For this review, take the finished solid that the model builds, in its own axes (mm). Coordinates: 2 decimals unless noted, no trailing zeros. Order: outer loops, then holes, each group sorted by start corner. A loop starts at its lowest first (then second) coordinate and runs counter-clockwise, first axis right, second up. Notation, with made-up numbers: (77.25, 73.25) -> (99.25, 73.25) arc R30 ccw to (99.25, 105.25) -> close; hole circle Ø4 at (10.5, -11). An arc over 180 degrees is marked (long way). Return JSON: item names as keys, results as strings. Group by question number.
Item 1: Take a section at D-D (x = 7.5). Write out the cut boundary in (y, z).
Item 2: For line 1 along Y through (x, z) = (22.5, -9.75); line 2 along X through (y, z) = (9, -10); line 3 along Y through (x, z) = (21.75, -9.5), list the stretches that pass through material, from the lowest coordinate up.
Item 3: Take a section at B-B (y = 10). Write out the cut boundary in (x, z), then the cut area to 3 significant figures.
Item 4: Insertion check: pin 1 (5 mm diameter, centred on x = 19.5, y = 8, fed in from +Z). The pin has a flat end and moves straight along its axis. Give the tip position at first contact, or say it passes through.
Item 5: Take a section at A-A (z = -20). Write out the cut boundary in (x, y).
Item 6: Take a section at C-C (x = 22.5). Write out the cut boundary in (y, z), then the cut area to 3 significant figures.
Item 7: Draft analysis for pull direction X (two halves, no side actions). For faces 1 (the flat face through (15, 20, -15)), 2 (the flat face through (0, 10, -15)), 3 (the cylindrical face through (5.94, 9.86, -20.35)), 4 (the flat face through (30, 10, -15)), state which applies: +X half, -X half, draft (parallel to the pull), parting line (faces both ways), or undercut.
```python
from build123d import *

# Parameters (mm, degrees)
SKETCH_1_W          = 30
SKETCH_1_H          = 30
SKETCH_1_R          = 1.6
EXTRUDE_1_DEPTH     = 20
SKETCH_2_R          = 1.6
CUT_EXTRUDE_1_DEPTH = 47.904157598


with BuildPart() as part:
    # 草图1 → 凸台-拉伸1 (new body)
    with BuildSketch(Plane(origin=(0, 0, 0), x_dir=(1, 0, 0), z_dir=(0, 1, 0))):
        with Locations((15, 15)):
            Rectangle(SKETCH_1_W, SKETCH_1_H)
        with Locations(Location((7.5, 20, 0), (0, 0, 270))):
            Circle(SKETCH_1_R, mode=Mode.SUBTRACT)
        with Locations(Location((7.5, 10, 0), (0, 0, 270))):
            Circle(SKETCH_1_R, mode=Mode.SUBTRACT)
    extrude(amount=EXTRUDE_1_DEPTH)

    # 草图2 → 切除-拉伸1 (cut, through all)
    with BuildSketch(Plane(origin=(0, 0, -30), x_dir=(-1, 0, 0), z_dir=(0, 0, -1))):
        with Locations((-22.5, 10)):
            Circle(SKETCH_2_R)
    extrude(amount=-CUT_EXTRUDE_1_DEPTH, mode=Mode.SUBTRACT)


solid = part.part
```
Findings below:
{
 "1": {"outline": "(0, -30) -> (20, -30) -> (20, -21.6) -> (0, -21.6) -> close; (0, -18.4) -> (20, -18.4) -> (20, -11.6) -> (0, -11.6) -> close; (0, -8.4) -> (20, -8.4) -> (20, 0) -> (0, 0) -> close"},
 "2": {"line 1": "y = 0 to 8.4, 11.6 to 20", "line 2": "x = 0 to 5.9, 9.1 to 21.25, 23.75 to 30", "line 3": "y = 0 to 8.59, 11.41 to 20"},
 "3": {"outline": "(0, -30) -> (20.9, -30) -> (20.9, 0) -> (0, 0) -> close; (24.1, -30) -> (30, -30) -> (30, 0) -> (24.1, 0) -> close; hole circle Ø3.2 at (7.5, -20); hole circle Ø3.2 at (7.5, -10)", "area": "788 mm2"},
 "4": {"pin 1": "stops at z = 0"},
 "5": {"outline": "(0, 0) -> (5.9, 0) -> (5.9, 20) -> (0, 20) -> close; (9.1, 0) -> (30, 0) -> (30, 20) -> (9.1, 20) -> close; hole circle Ø3.2 at (22.5, 10)"},
 "6": {"outline": "(0, -30) -> (8.4, -30) -> (8.4, 0) -> (0, 0) -> close; (11.6, -30) -> (20, -30) -> (20, 0) -> (11.6, 0) -> close", "area": "504 mm2"},
 "7": {"face 1": "draft", "face 2": "-X half", "face 3": "undercut", "face 4": "+X half"}
}
